The model under review builds one solid part; all positions refer to its coordinate system, in mm. A direction names the side the tool comes from. Give positions to 0.01 mm unless a question says otherwise; leave off trailing zeros. Write each loop counter-clockwise with the first axis right and the second up, starting at its lowest first coordinate (ties: lowest second). Pieces come first, ordered by that corner, then holes. Notation, with made-up numbers: (18, 14.25) - (59, 14.25) arc R25 ccw to (59, 42.25) - close; hole circle Ø1 at (15.25, 52). An arc over 180 degrees is marked (long way). One line per question, with ' | ' between items. Start each with the question number.
Autodesk Inventor part; units mm, degrees
ref_plane "YZ Plane" through (0, 0, 0) normal (1, 0, 0) x (0, 1, 0)
ref_plane "XZ Plane" through (0, 0, 0) normal (0, 1, 0) x (-1, 0, 0)
ref_plane "XY Plane" through (0, 0, 0) normal (0, 0, 1) x (1, 0, 0)
sketch "Sketch1" plane through (0, 0, 0) normal (0, 1, 0) x (-1, 0, 0)
  circle A0 centre (0, 0) radius 12.5
  dimension "d0" = 25
extrude "Extrusion1" add sketch "Sketch1" along normal blind 50
sketch "Sketch2" plane through (0, 50, 0) normal (0, 1, 0) x (1, 0, 0)
  circle A0 centre (0, 0) radius 3.5
  dimension "d3" = 7
extrude "Extrusion2" add sketch "Sketch2" along normal blind 2.5
sketch "Sketch3" plane through (0, 52.5, 0) normal (0, 1, 0) x (1, 0, 0)
  circle A0 centre (0, 0) radius 2
  dimension "d6" = 4
extrude "Extrusion3" add sketch "Sketch3" along normal blind 8
sketch "Sketch4" plane through (0, 0, 0) normal (0, -1, 0) x (1, 0, 0)
  circle A0 centre (0, 0) radius 7
  dimension "d9" = 14
extrude "Extrusion4" add sketch "Sketch4" along normal blind 9
sketch "Sketch5" plane through (0, 50, 0) normal (0, 1, 0) x (1, 0, 0)
  circle A0 centre (0, 0) radius 3.5
  point P0 (-8.382, 0)
  point P1 (8.382, 0)
  dimension "d12" = 8.382
  dimension "d13" = 8.382
hole "Hole1" at (-8.382, 50, 0) at (8.382, 50, 0) direction (0, -1, 0) diameter 2.4638 depth 8.7884
properties part number "Motor"
Item 1: Take a section at D-D (x = 4.75). Give the boundary of the cut face in (y, z).
Item 2: Take a section at C-C (y = 53.5). Give the boundary of the cut face in (x, z).
Item 3: Clearance check with flat-ended pins moving along their axes: P1, Ø2, axis at y = 49.5, z = 1.5, coming from the +X side; P2, Ø1.5, axis at y = 39, z = -8.5, coming from the -X side; P3, Ø2, axis at x = -8, z = 0.5, coming from the +Y side. State where each tip first meets the part, or that it passes through.
Item 4: Take a section at A-A (z = 0). Give the boundary of the cut face in (x, y).
Item 5: Take a section at B-B (x = 0). Give the boundary of the cut face in (y, z).
Item 6: For probe 1 along Y at (x, z) = (8, 6); probe 2 along Y at (x, z) = (2.25, 3); probe 3 along X at (y, z) = (14, -10), list the stretches that pass through material, from the lowest coordinate up.
Item 7: Machinability: for faces 1 (the cylindrical face through (6.466, -4.437, 2.681)), 2 (the flat face through (0, 60.5, 0)), 3 (the cylindrical face through (9.585, 45.544, -0.267)), which of the approach directions +Z, -Z, +X, -X, +Y, -Y give a long, thin tool a straight path to every point of the face, cutting with its end or side? Answer none if there is none.
Check sheet entries:
1) outline: (-9, -5.14) - (0, -5.14) - (0, -11.56) - (50, -11.56) - (50, 11.56) - (0, 11.56) - (0, 5.14) - (-9, 5.14) - close
2) outline: circle Ø4 at (0, 0)
3) P1: stops at x = 12.49 | P2: stops at x = -9.81 | P3: stops at y = 50
4) outline: (-12.5, 0) - (-7, 0) - (-7, -9) - (7, -9) - (7, 0) - (12.5, 0) - (12.5, 50) - (9.61, 50) - (9.61, 41.21) - (7.15, 41.21) - (7.15, 50) - (3.5, 50) - (3.5, 52.5) - (2, 52.5) - (2, 60.5) - (-2, 60.5) - (-2, 52.5) - (-3.5, 52.5) - (-3.5, 50) - (-7.15, 50) - (-7.15, 41.21) - (-9.61, 41.21) - (-9.61, 50) - (-12.5, 50) - close
5) outline: (-9, -7) - (0, -7) - (0, -12.5) - (50, -12.5) - (50, -3.5) - (52.5, -3.5) - (52.5, -2) - (60.5, -2) - (60.5, 2) - (52.5, 2) - (52.5, 3.5) - (50, 3.5) - (50, 12.5) - (0, 12.5) - (0, 7) - (-9, 7) - close
6) probe 1: y = 0 to 50 | probe 2: y = -9 to 50 | probe 3: x = -7.5 to 7.5
7) face 1: -Y | face 2: +Z, -Z, +X, -X, +Y | face 3: +Y
